from build123d import *

# Parameters (mm, degrees)
BOX_W           = 15
BOX_H           = 15
BOX_DEPTH       = 15
SKETCH_W        = 110
SKETCH_H        = 80
PAD_DEPTH       = 5
SKETCH001_R     = 2.1
POCKET_DEPTH    = 5
CHAMFER_SIZE    = 1
SKETCH002_W     = 89
SKETCH002_H     = 2
SKETCH002_W_2   = 2
SKETCH002_H_2   = 59
PAD001_DEPTH    = 5
CHAMFER001_SIZE = 1
FILLET_R        = 2


with BuildPart() as cube:
    # Box → Box (new body)
    with BuildSketch(Plane(origin=(40, 25, 0), x_dir=(1, 0, 0), z_dir=(0, 0, 1))):
        with Locations((7.5, 7.5)):
            Rectangle(BOX_W, BOX_H)
    extrude(amount=BOX_DEPTH)


with BuildPart() as common:
    # Sketch → Pad (new body)
    with BuildSketch(Plane.XY):
        Rectangle(SKETCH_W, SKETCH_H)
    extrude(amount=PAD_DEPTH)

    # Sketch001 (on Face6 of Pad) → Pocket (cut)
    with BuildSketch(Plane.XY.offset(5)):
        with Locations((49, 34)):
            Circle(SKETCH001_R)
        with Locations((-49, 34)):
            Circle(SKETCH001_R)
        with Locations((-49, -34)):
            Circle(SKETCH001_R)
        with Locations((49, -34)):
            Circle(SKETCH001_R)
    extrude(amount=-POCKET_DEPTH, mode=Mode.SUBTRACT)

    # Chamfer
    chamfer_edges = [common.edges().sort_by_distance(p)[0] for p in [
        (-51.1, -34, 0),
        (-51.1, 34, 0),
        (46.9, 34, 0),
        (46.9, -34, 0),
    ]]
    chamfer(chamfer_edges, length=CHAMFER_SIZE)

    # Sketch002 (on Face11 of Chamfer) → Pad001 (join)
    with BuildSketch(Plane.XY.offset(5)):
        with Locations((0, 36.5)):
            Rectangle(SKETCH002_W, SKETCH002_H)
        with Locations((0, -36.5)):
            Rectangle(SKETCH002_W, SKETCH002_H)
        with Locations((51.5, 0)):
            Rectangle(SKETCH002_W_2, SKETCH002_H_2)
        with Locations((-51.5, 0)):
            Rectangle(SKETCH002_W_2, SKETCH002_H_2)
    extrude(amount=PAD001_DEPTH)

    # Chamfer001
    chamfer001_edges = [common.edges().sort_by_distance(p)[0] for p in [
        (-52.5, 0, 10),
        (0, 37.5, 10),
        (52.5, 0, 10),
        (0, -37.5, 10),
    ]]
    chamfer(chamfer001_edges, length=CHAMFER001_SIZE)

    # Fillet
    fillet_edges = [common.edges().sort_by_distance(p)[0] for p in [
        (-55, -40, 2.5),
        (-55, 0, 0),
        (-55, 40, 2.5),
        (0, 40, 0),
        (55, 40, 2.5),
        (55, 0, 0),
        (55, -40, 2.5),
        (0, -40, 0),
    ]]
    fillet(fillet_edges, radius=FILLET_R)

    # Common: intersect Cube
    add(cube.part, mode=Mode.INTERSECT)


solid = common.part
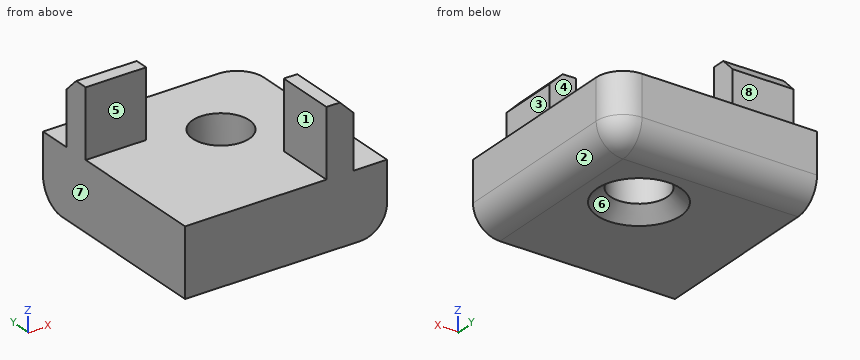
Geometry check sheet. Reference: the model listing, model coordinates, mm. Face numbers are marked on the shaded views. A direction names the side the tool comes from. Round coordinates to 2 decimals unless told otherwise and drop trailing zeros. Write each loop counter-clockwise with the first axis right and the second up, starting at its lowest first coordinate (ties: lowest second). Pieces come first, ordered by that corner, then holes. Notation, with made-up numbers: (52.25, 79) -> (107.25, 79) arc R36 cw to (107.25, 114) -> close; hole circle Ø6 at (-37.5, -10.5). An arc over 180 degrees is marked (long way). One line per item, written item: value. Start each with the question number.
(1) Access from +Z, -Z, +X, -X, +Y, -Y to the whole of each face (thin tool, end or side, straight path). Record for the marked faces 1, 2, 3, 4 and 5.
(2) Scan lines: line 1 (Y direction, x = 49, z = 3.1); line 2 (Z direction, x = 46, y = 28.25); line 3 (X direction, y = 26.5, z = 6.5). Record each from-to range of solid material in increasing order. Write a range as [from, to].
(3) Draft check along X on the marked faces 6, 7 and 8. Enter one of: +X half, -X half, draft (parallel to the pull), parting line (faces both ways), or undercut.
(4) Cross-section at C-C, the plane z = 7. Record the cut outline in (x, y).
(5) Cross-section at D-D, the plane z = 1.25. Record the cut outline in (x, y).
(6) Cross-section at A-A, the plane y = 34. Record the cut outline in (x, z), and give its area (3 significant figures).
(7) Go/stop test with flat-tipped pins: pin 1 Ø2 at (x, z) = (51, 6.5) entering from +Y; pin 2 Ø5 at (y, z) = (26.5, 6.5) entering from -X; pin 3 Ø0.6 at (y, z) = (36.5, 8.5) entering from +X; pin 4 Ø2 at (y, z) = (26.5, 7.5) entering from +X. Record where each tip stops, or that it passes through.
(8) Cross-section at B-B, the plane x = 49. Record the cut outline in (y, z), and give its area (3 significant figures).
Answer:
1. face 1: +Z, -X, +Y, -Y
1. face 2: -Z, +X, +Y, -Y
1. face 3: +Z, +X, +Y, -Y
1. face 4: +Z, +X, -X, +Y
1. face 5: +Z, +X, -X, -Y
2. line 1: [25, 31.9], [36.1, 40]
2. line 2: [0, 5]
2. line 3: [50.5, 52.5]
3. face 6: undercut
3. face 7: -X half
3. face 8: draft
4. outline: (40, 35.5) -> (44.5, 35.5) -> (44.5, 37.5) -> (40, 37.5) -> close; (50.5, 25) -> (52.5, 25) -> (52.5, 29.5) -> (50.5, 29.5) -> close
5. outline: (40, 25) -> (54.85, 25) -> (54.85, 38) arc R1.85 ccw to (53, 39.85) -> (40, 39.85) -> close; hole circle Ø4.2 at (49, 34)
6. outline: (40, 0) -> (45.9, 0) -> (46.9, 1) -> (46.9, 5) -> (40, 5) -> close; (51.1, 1) -> (52.1, 0) -> (53, 0) arc R2 ccw to (55, 2) -> (55, 5) -> (51.1, 5) -> close
6. area: 52.1 mm²
7. pin 1: y = 29.5
7. pin 2: x = 40
7. pin 3: x = 44.5
7. pin 4: x = 52.5
8. outline: (25, 0) -> (30.9, 0) -> (31.9, 1) -> (31.9, 5) -> (25, 5) -> close; (36.1, 1) -> (37.1, 0) -> (38, 0) arc R2 ccw to (40, 2) -> (40, 5) -> (36.1, 5) -> close
8. area: 52.1 mm²
